```python
from build123d import *

# Parameters (mm, degrees)
SKETCH1_W            = 50
SKETCH1_H            = 126
BOSS_EXTRUDE1_DEPTH  = 0.99736772
SKETCH2_W            = 40
SKETCH2_H            = 3
BOSS_EXTRUDE2_DEPTH  = 0.1
SKETCH6_W            = 52
SKETCH6_H            = 128
SKETCH6_W_2          = 50
SKETCH6_H_2          = 126
BOSS_EXTRUDE8_DEPTH  = 1.4
SKETCH11_W           = 40
SKETCH11_H           = 3
BOSS_EXTRUDE12_DEPTH = 0.1
SKETCH12_W           = 40
SKETCH12_H           = 3
BOSS_EXTRUDE13_DEPTH = 0.1
SKETCH13_W           = 40
SKETCH13_H           = 3
BOSS_EXTRUDE14_DEPTH = 0.1
SKETCH14_W           = 40
SKETCH14_H           = 3
BOSS_EXTRUDE15_DEPTH = 0.1


with BuildPart() as part:
    # Sketch1 → Boss-Extrude1 (new body)
    with BuildSketch(Plane(origin=(0, 0, 0), x_dir=(1, 0, 0), z_dir=(0, 1, 0))):
        with Locations((-71.774193548, -38.230414747)):
            Rectangle(SKETCH1_W, SKETCH1_H)
    extrude(amount=BOSS_EXTRUDE1_DEPTH)

    # Sketch2 → Boss-Extrude2 (add)
    with BuildSketch(Plane(origin=(0, 0.99736772, 0), x_dir=(1, 0, 0), z_dir=(0, 1, 0))):
        with Locations((-71.774193548, 18.269585253)):
            Rectangle(SKETCH2_W, SKETCH2_H)
        with Locations((-71.774193548, 5.269585253)):
            Rectangle(SKETCH2_W, SKETCH2_H)
    extrude(amount=BOSS_EXTRUDE2_DEPTH)

    # Sketch6 → Boss-Extrude8 (add)
    with BuildSketch(Plane(origin=(0, 0, 0), x_dir=(1, 0, 0), z_dir=(0, 1, 0))):
        with Locations((-71.921181358, -38.105868157)):
            Rectangle(SKETCH6_W, SKETCH6_H)
        with Locations((-71.774193548, -38.230414747)):
            Rectangle(SKETCH6_W_2, SKETCH6_H_2, mode=Mode.SUBTRACT)
    extrude(amount=BOSS_EXTRUDE8_DEPTH)

    # Sketch11 → Boss-Extrude12 (add)
    with BuildSketch(Plane(origin=(0, 0.99736772, 0), x_dir=(1, 0, 0), z_dir=(0, 1, 0))):
        with Locations((-71.666893543, -5.127021843)):
            Rectangle(SKETCH11_W, SKETCH11_H)
        with Locations((-71.666893543, -18.127021843)):
            Rectangle(SKETCH11_W, SKETCH11_H)
    extrude(amount=BOSS_EXTRUDE12_DEPTH)

    # Sketch12 → Boss-Extrude13 (add)
    with BuildSketch(Plane(origin=(0, 0.99736772, -2.5), x_dir=(1, 0, 0), z_dir=(0, 1, 0))):
        with Locations((-71.666893543, -30.328159375)):
            Rectangle(SKETCH12_W, SKETCH12_H)
        with Locations((-71.666893543, -43.328159375)):
            Rectangle(SKETCH12_W, SKETCH12_H)
    extrude(amount=BOSS_EXTRUDE13_DEPTH)

    # Sketch13 → Boss-Extrude14 (add)
    with BuildSketch(Plane(origin=(0, 0.99736772, 0), x_dir=(1, 0, 0), z_dir=(0, 1, 0))):
        with Locations((-71.498865442, -55.766480825)):
            Rectangle(SKETCH13_W, SKETCH13_H)
        with Locations((-71.498865442, -68.766480825)):
            Rectangle(SKETCH13_W, SKETCH13_H)
    extrude(amount=BOSS_EXTRUDE14_DEPTH)

    # Sketch14 → Boss-Extrude15 (add)
    with BuildSketch(Plane(origin=(0, 0.99736772, 0), x_dir=(1, 0, 0), z_dir=(0, 1, 0))):
        with Locations((-71.677348389, -80.754093343)):
            Rectangle(SKETCH14_W, SKETCH14_H)
        with Locations((-71.677348389, -93.754093343)):
            Rectangle(SKETCH14_W, SKETCH14_H)
    extrude(amount=BOSS_EXTRUDE15_DEPTH)


solid = part.part
```
Can you work these out from the model? Positions are in its coordinate system, mm. A direction names the side the tool comes from. Coordinates: 2 decimals unless noted, no trailing zeros. Write each loop counter-clockwise with the first axis right and the second up, starting at its lowest first coordinate (ties: lowest second). Pieces come first, ordered by that corner, then holes. Notation, with made-up numbers: M 19.25,-25 L 69.25,-25 A25 ccw 69.25,-3 Z; hole C 28,1.25 d9. An arc over 180 degrees is marked long. Write item = value, one per line. Start each with the question number.
Q1. On a 3-axis mill with a long thin cutter (end or side, diameter ignored), from which of +Z, -Z, +X, -X, +Y, -Y can I reach the whole of each face in a straight line? I mean faces 3 (the face through (-72, 1.097, -18)), 4 (the face through (-97, 1.4, 38)). Say none if no direction works.
Q2. If I drill on L1, parallel to Z at x = -88, y = 1.35; L2, parallel to X at y = 1.35, z = -5; L3, parallel to Y at x = -59.5, z = 49.5, over which ranges is the centre line in solid material (lowest first)? Write a range as [from, to].
Q3. Thinking about a two-plate mould opening in X: for faces 1 (the face through (-72, 0, 37)), 2 (the face through (-72, 1.097, 41)), which applies, released by +X, released by -X, zero draft, split by the parting line, or undercut?
Q4. If we section it at B-B, the plane z = -13.5: Write out the boundary of the cut face in (x, y), then the cut area to 3 significant figures.
Q5. If we section it at A-A, the plane x = -49: Write out the boundary of the cut face in (y, z), then the cut area to 3 significant figures.
Q6. I'm going to push flat-ended pins straight in: pin 1 (3 mm diameter, centred on x = -88.5, z = 44, fed in from +Y); pin 2 (1.5 mm diameter, centred on x = -54.5, z = 87.5, fed in from -Y); pin 3 (1.5 mm diameter, centred on x = -80, z = 80.5, fed in from +Y). Where does each tip first touch, or does it pass through?
Check sheet entries:
q1.face_3 = +Y
q1.face_4 = +Z, -Z, +X, -X, +Y
q2.L1 = [-25.89, -24.77], [101.23, 102.11]
q2.L2 = [-97.92, -96.77], [-46.77, -45.92]
q2.L3 = [0, 1]
q3.face_1 = zero draft
q3.face_2 = undercut
q4.outline = M -97.92,0 L -45.92,0 L -45.92,1.4 L -46.77,1.4 L -46.77,1 L -96.77,1 L -96.77,1.4 L -97.92,1.4 Z
q4.area = 52.7 mm²
q5.outline = M 0,-25.89 L 1.4,-25.89 L 1.4,-24.77 L 1,-24.77 L 1,101.23 L 1.4,101.23 L 1.4,102.11 L 0,102.11 Z
q5.area = 128 mm²
q6.pin_1 = 1
q6.pin_2 = 0
q6.pin_3 = 1.1
